```python
from build123d import *

# Parameters (mm, degrees)
SKIZZE1_W                            = 54.7
SKIZZE1_H                            = 6
SKIZZE2_W                            = 10
SKIZZE2_H                            = 20
SCHNITT_LINEAR_AUSTRAGEN1_DEPTH      = 12
SCHNITT_LINEAR_AUSTRAGEN1_DEPTH_BACK = 12


with BuildPart() as part:
    # Skizze1 → Rotation1 (revolve)
    with BuildSketch(Plane.XY):
        with Locations((21.25, 3)):
            Rectangle(SKIZZE1_W, SKIZZE1_H)
    revolve(axis=Axis((48.6, 0, 0), (-1, 0, 0)))

    # Skizze2 → Rotation2 (revolve)
    with BuildSketch(Plane.XY):
        with Locations((43.6, 10)):
            Rectangle(SKIZZE2_W, SKIZZE2_H)
    revolve(axis=Axis((48.6, 0, 0), (-1, 0, 0)))

    # Skizze3 → Schnitt-Linear austragen1 (cut, two sides)
    with BuildSketch(Plane.XY) as schnitt_linear_austragen1_sk:
        Polygon((-36.2, -16), (4.950852961, -16), (-1.4, -5), (-6.1, -5), (-6.1, -10), (-30.1, -10), (-30.1, 10), (-6.1, 10), (-6.1, 5), (-1.4, 5), (4.950852961, 16), (-36.2, 16), align=None)
    extrude(amount=SCHNITT_LINEAR_AUSTRAGEN1_DEPTH, mode=Mode.SUBTRACT)
    extrude(schnitt_linear_austragen1_sk.sketch, amount=-SCHNITT_LINEAR_AUSTRAGEN1_DEPTH_BACK, mode=Mode.SUBTRACT)

    # Skizze4 → Schnitt-Rotation1 (revolve, cut)
    with BuildSketch(Plane.XY):
        Polygon((-6.1, 0), (-6.1, 4.8), (-5.5, 4.2), (-2.8, 4.2), (-2.8, 4), (-2.1235, 3.3235), (13.9, 3.3235), (15.81882362, 0), align=None)
    revolve(axis=Axis((15.81882362, 0, 0), (-1, 0, 0)), mode=Mode.SUBTRACT)


solid = part.part
```
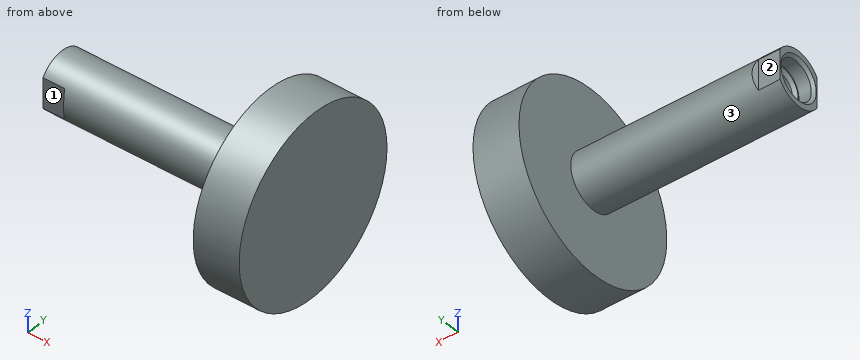
CAD build for the part. Positions are in the model's coordinates, mm. Face numbers are marked on the shaded views. A direction names the side the tool comes from. Round coordinates to 2 decimals unless told otherwise and drop trailing zeros. Loops run counter-clockwise (first coordinate to the right, second up) from the corner with the lowest first, then second, coordinate; pieces in that order, holes last. Notation, with made-up numbers: (53.5, 71) - (90.5, 71) arc R21 cw to (90.5, 108) - close; hole circle Ø10 at (88, 58.25). An arc over 180 degrees is marked (long way). Return JSON: item names as keys, results as strings. Group by question number.
Q1. Band-saw the part on B-B on y = -9.5. Give the cut face in (x, z), plus the area to 3 significant figures.
Q2. Flat gauge pins, fed straight in: pin 1 Ø10 at (x, z) = (31.5, 5.5) entering from +Y; pin 2 Ø4 at (x, y) = (18.5, -3) entering from +Z; pin 3 Ø2 at (y, z) = (-4.5, -16) entering from -X. Where does each tip first touch, or does it go through?
Q3. Tool access for the marked faces 1, 2 and 3: list every direction of +Z, -Z, +X, -X, +Y, -Y with a clear straight run to the whole face (end or side of a thin tool).
Q4. Band-saw the part on A-A on x = 43.5. Give the cut face in (y, z).
Q5. Band-saw the part on C-C on z = 11.5. Give the cut face in (x, y).
Q6. Band-saw the part on D-D on x = 34. Give the cut face in (y, z), plus the area to 3 significant figures.
Q7. Drill centre lines: line 1 along Z through (x, y) = (-3, 0); line 2 along Y through (x, z) = (1, 0); line 3 along X through (y, z) = (-12, 12.5). Where is each one in solid material? Low to high. Write a range as [from, to].
Solutions:
{
 "1": {"outline": "(38.6, -17.6) - (48.6, -17.6) - (48.6, 17.6) - (38.6, 17.6) - close", "area": "352 mm^2"},
 "2": {"pin 1": "stops at y = 5.98", "pin 2": "stops at z = 5.92", "pin 3": "stops at x = 38.6"},
 "3": {"face 1": "+Z, -Z, -X, -Y", "face 2": "+Z, -Z, -X, +Y", "face 3": "-X"},
 "4": {"outline": "circle Ø40 at (0, 0)"},
 "5": {"outline": "(38.6, -16.36) - (48.6, -16.36) - (48.6, 16.36) - (38.6, 16.36) - close"},
 "6": {"outline": "circle Ø12 at (0, 0)", "area": "113 mm^2"},
 "7": {"line 1": "z = [-6, -4.2], [4.2, 6]", "line 2": "y = [-6, -3.32], [3.32, 6]", "line 3": "x = [38.6, 48.6]"}
}
